For this review, take the finished solid that the model builds, in its own axes (mm). A direction names the side the tool comes from. Give positions to 0.01 mm unless a question says otherwise; leave off trailing zeros. Order: outer loops, then holes, each group sorted by start corner. A loop starts at its lowest first (then second) coordinate and runs counter-clockwise, first axis right, second up. Notation, with made-up numbers: (21, -11) -> (32, -11) arc R19 ccw to (32, 19) -> close; hole circle Ø8 at (-8, 19). An arc over 180 degrees is marked (long way). Return JSON: item names as keys, results as strings. Group by question number.
1) Add section B-B (y = 5). Give the boundary of the cut face in (x, z).
2) To check wall thickness, follow line 1 along Y through (x, z) = (0, -0.5); line 2 along X through (y, z) = (16.5, -5.75); line 3 along Z through (x, y) = (-29.5, -7.5). State the ranges of each line that lie inside material, in increasing order.
3) Insertion check: P1, Ø1, axis at x = -30, z = -2.5, coming from the +Y side; P2, Ø3, axis at y = 5.5, z = -4, coming from the +X side; P3, Ø3.5, axis at y = 16.5, z = -3.5, coming from the +X side; P4, Ø0.5, axis at x = -39.5, z = -1, coming from the +Y side. Each pin has a flat end and moves straight along its axis. Give the tip position at first contact, or say it passes through.
4) Add section C-C (z = -6). Give the boundary of the cut face in (x, y).
5) Add section A-A (x = 26). Give the boundary of the cut face in (y, z), then the cut area to 3 significant figures.
6) Add section D-D (x = -26). Give the boundary of the cut face in (y, z).
7) For faces 1 (the face through (20, 17, -1.9)), 2 (the face through (-20, 17, -1.9)), 3 (the face through (10, 14, -3.5)), list the 3-axis set-ups (+Z, -Z, +X, -X, +Y, -Y) from which the entire face can be reached by the end or side of a thin tool; tool diameter is ignored.
8) The part is to be moulded in two halves that separate along Z. For faces 4 (the face through (10.367, 17.595, -4.525)), 5 (the face through (-27.84, 6.69, -0.89)), 6 (the face through (-1, -1, 0)), say which applies: released by +Z, released by -Z, zero draft, split by the parting line, or undercut.
from build123d import *

# Parameters (mm, degrees)
SKETCH2_W             = 80
SKETCH2_H             = 40
BASE_FLANGE1_DEPTH    = 2
HEM1_START            = -40
HEM1_DEPTH            = 21
HEM1_2_DEPTH          = 1
HEM1_START_2          = -20
HEM1_3_DEPTH          = 1
HEM1_START_3          = -39
HEM1_4_DEPTH          = 19
HEM3_DEPTH            = 21
HEM3_2_DEPTH          = 1
HEM3_START            = 20
HEM3_3_DEPTH          = 1
HEM3_START_2          = 1
HEM3_4_DEPTH          = 19
CUT_EXTRUDE1_REACH    = 47
SKETCH13_W            = 1
SKETCH13_H            = 2.753292139
FILLET1_R             = 5
F_5_0MM_DOWEL_HOLE1_D = 5
CHAMFER1_SIZE         = 0.2


# Read off the part's stored shape, not the designer's step: Hem1, Hem3
# Sheet-metal steps are written as plain solids
with BuildPart() as part:
    # Sketch2 → Base-Flange1 (new body)
    with BuildSketch(Plane.XY):
        Rectangle(SKETCH2_W, SKETCH2_H)
    extrude(amount=-BASE_FLANGE1_DEPTH)

    # Hem1 outline → Hem1 (cut)
    with BuildSketch(Plane.YZ.offset(HEM1_START)):
        with BuildLine():
            Line((20, 0), (16.5, 0))
            ThreePointArc((16.5, 0), (18.370828693, -0.541960108), (19.66227766, -2))
            Line((19.66227766, -2), (20, -2))
            Line((20, -2), (20, 0))
        make_face()
    extrude(amount=HEM1_DEPTH, mode=Mode.SUBTRACT)

    # Hem1 2 outline → Hem1 2 (cut)
    with BuildSketch(Plane.YZ.offset(HEM1_START)):
        with BuildLine():
            Line((15.5, 0), (15.5, -2))
            Line((15.5, -2), (19.66227766, -2))
            ThreePointArc((19.66227766, -2), (18.370828693, -0.541960108), (16.5, 0))
            Line((16.5, 0), (15.5, 0))
        make_face()
    extrude(amount=HEM1_2_DEPTH, mode=Mode.SUBTRACT)

    # Hem1 3 outline → Hem1 3 (cut)
    with BuildSketch(Plane.YZ.offset(HEM1_START_2)):
        with BuildLine():
            Line((15.5, 0), (15.5, -2))
            Line((15.5, -2), (19.66227766, -2))
            ThreePointArc((19.66227766, -2), (18.370828693, -0.541960108), (16.5, 0))
            Line((16.5, 0), (15.5, 0))
        make_face()
    extrude(amount=HEM1_3_DEPTH, mode=Mode.SUBTRACT)

    # Hem1 4 outline → Hem1 4 (add)
    with BuildSketch(Plane.YZ.offset(HEM1_START_3)):
        with BuildLine():
            Line((19.66227766, -2), (16.5, -2))
            ThreePointArc((16.5, -2), (17.560660172, -4.560660172), (15, -3.5))
            Line((15, -3.5), (13, -3.5))
            ThreePointArc((13, -3.5), (17.268774411, -6.914525722), (19.66227766, -2))
        make_face()
    extrude(amount=HEM1_4_DEPTH)

    # Hem3 outline → Hem3 (cut)
    with BuildSketch(Plane.YZ):
        with BuildLine():
            Line((20, 0), (16.5, 0))
            ThreePointArc((16.5, 0), (18.370828693, -0.541960108), (19.66227766, -2))
            Line((19.66227766, -2), (20, -2))
            Line((20, -2), (20, 0))
        make_face()
    extrude(amount=HEM3_DEPTH, mode=Mode.SUBTRACT)

    # Hem3 2 outline → Hem3 2 (cut)
    with BuildSketch(Plane.YZ):
        with BuildLine():
            Line((15.5, 0), (15.5, -2))
            Line((15.5, -2), (19.66227766, -2))
            ThreePointArc((19.66227766, -2), (18.370828693, -0.541960108), (16.5, 0))
            Line((16.5, 0), (15.5, 0))
        make_face()
    extrude(amount=HEM3_2_DEPTH, mode=Mode.SUBTRACT)

    # Hem3 3 outline → Hem3 3 (cut)
    with BuildSketch(Plane.YZ.offset(HEM3_START)):
        with BuildLine():
            Line((15.5, 0), (15.5, -2))
            Line((15.5, -2), (19.66227766, -2))
            ThreePointArc((19.66227766, -2), (18.370828693, -0.541960108), (16.5, 0))
            Line((16.5, 0), (15.5, 0))
        make_face()
    extrude(amount=HEM3_3_DEPTH, mode=Mode.SUBTRACT)

    # Hem3 4 outline → Hem3 4 (add)
    with BuildSketch(Plane.YZ.offset(HEM3_START_2)):
        with BuildLine():
            Line((19.66227766, -2), (16.5, -2))
            ThreePointArc((16.5, -2), (17.560660172, -4.560660172), (15, -3.5))
            Line((15, -3.5), (13, -3.5))
            ThreePointArc((13, -3.5), (17.268774411, -6.914525722), (19.66227766, -2))
        make_face()
    extrude(amount=HEM3_4_DEPTH)

    # Sketch13 → Cut-Extrude1 (cut, up to next)
    with BuildSketch(Plane(origin=(0, 0, -2), x_dir=(-1, 0, 0), z_dir=(0, 0, -1)), mode=Mode.PRIVATE) as cut_extrude1_sk1:
        Polygon((-21, 12.5), (-40, 12.5), (-40, 20), (-21, 20), (-21, 15.5), (-20, 15.5), (-20, 12.5), align=None)
    cut_extrude1_tool1 = extrude(cut_extrude1_sk1.sketch, amount=-CUT_EXTRUDE1_REACH, mode=Mode.PRIVATE) & part.part
    # Sketch13 → Cut-Extrude1 (cut, up to next)
    with BuildSketch(Plane(origin=(0, 0, -2), x_dir=(-1, 0, 0), z_dir=(0, 0, -1)), mode=Mode.PRIVATE) as cut_extrude1_sk2:
        Polygon((19, 12.5), (0, 12.5), (-1, 12.5), (-1, 15.5), (0, 15.5), (0, 20), (19, 20), (19, 15.5), (20, 15.5), (20, 12.5), align=None)
    cut_extrude1_tool2 = extrude(cut_extrude1_sk2.sketch, amount=-CUT_EXTRUDE1_REACH, mode=Mode.PRIVATE) & part.part
    # Sketch13 → Cut-Extrude1 (cut, up to next)
    with BuildSketch(Plane(origin=(0, 0, -2), x_dir=(-1, 0, 0), z_dir=(0, 0, -1)), mode=Mode.PRIVATE) as cut_extrude1_sk3:
        with Locations((39.5, 14.123353931)):
            Rectangle(SKETCH13_W, SKETCH13_H)
    cut_extrude1_tool3 = extrude(cut_extrude1_sk3.sketch, amount=-CUT_EXTRUDE1_REACH, mode=Mode.PRIVATE) & part.part
    add(cut_extrude1_tool1.solids().sort_by_distance((30.293814, 16.203608, -2))[0], mode=Mode.SUBTRACT)
    add(cut_extrude1_tool2.solids().sort_by_distance((-9.5, 16.159091, -2))[0], mode=Mode.SUBTRACT)
    add(cut_extrude1_tool3.solids().sort_by_distance((-39.5, 14.123354, -2))[0], mode=Mode.SUBTRACT)

    # Fillet1
    fillet1_edges = [part.edges().sort_by_distance(p)[0] for p in [
        (40, -20, -1),
        (-40, -20, -1),
    ]]
    fillet(fillet1_edges, radius=FILLET1_R)

    # Ø5.0mm Dowel Hole1 (through all)
    with Locations(Plane(origin=(0, 0, -2), x_dir=(-1, 0, 0), z_dir=(0, 0, -1))):
        with Locations((-26, 5), (26, 5), (0, -10)):
            Hole(F_5_0MM_DOWEL_HOLE1_D / 2)

    # Chamfer1
    chamfer1_edges = [part.edges().sort_by_distance(p)[0] for p in [
        (-2.5, -10, -2),
        (-28.5, 5, -2),
        (23.5, 5, -2),
    ]]
    chamfer(chamfer1_edges, length=CHAMFER1_SIZE)


solid = part.part
Evaluation:
{
 "1": {"outline": "(-40, -2) -> (-28.7, -2) -> (-28.5, -1.8) -> (-28.5, 0) -> (-40, 0) -> close; (-23.5, -1.8) -> (-23.3, -2) -> (23.3, -2) -> (23.5, -1.8) -> (23.5, 0) -> (-23.5, 0) -> close; (28.5, -1.8) -> (28.7, -2) -> (40, -2) -> (40, 0) -> (28.5, 0) -> close"},
 "2": {"line 1": "-20 to -12.5, -7.5 to 12.5", "line 2": "-39 to -20, 1 to 20", "line 3": "-2 to 0"},
 "3": {"P1": "y = 19.96", "P2": "through", "P3": "x = 20", "P4": "y = 12.75"},
 "4": {"outline": "(-39, 14.05) -> (-20, 14.05) -> (-20, 18.95) -> (-39, 18.95) -> close; (1, 14.05) -> (20, 14.05) -> (20, 18.95) -> (1, 18.95) -> close"},
 "5": {"outline": "(-20, -2) -> (2.3, -2) -> (2.5, -1.8) -> (2.5, 0) -> (-20, 0) -> close; (7.5, -1.8) -> (7.7, -2) -> (12.5, -2) -> (12.5, 0) -> (7.5, 0) -> close", "area": "55.0 mm^2"},
 "6": {"outline": "(-20, -2) -> (2.3, -2) -> (2.5, -1.8) -> (2.5, 0) -> (-20, 0) -> close; (7.5, -1.8) -> (7.7, -2) -> (16.5, -2) arc R1.5 cw (long way) to (15, -3.5) -> (13, -3.5) arc R3.5 ccw (long way) to (16.5, 0) -> (7.5, 0) -> close"},
 "7": {"face 1": "+Z, -Z, +X, +Y", "face 2": "+Z, -Z, +Y", "face 3": "+X, -X, -Y"},
 "8": {"face 4": "undercut", "face 5": "zero draft", "face 6": "released by +Z"}
}
